Geometry check sheet. Reference: the model listing, model coordinates, mm. A direction names the side the tool comes from. Give positions to 0.01 mm unless a question says otherwise; leave off trailing zeros. Write each loop counter-clockwise with the first axis right and the second up, starting at its lowest first coordinate (ties: lowest second). Pieces come first, ordered by that corner, then holes.
(1) Tool access check on faces 1 (the flat face through (41.686, -9, 5)), 2 (the flat face through (70, 4.42, 5)), 3 (the flat face through (8.02, -22, 5)), 4 (the flat face through (0, -38.015, 5)). Record the directions out of +Z, -Z, +X, -X, +Y, -Y that give a thin tool (end or side, any length) a straight path to the whole face; none if there is none.
(2) Cross-section at C-C (x = 29). Record the boundary of the cut face in (y, z), and give its area (3 significant figures).
(3) Thickness scan on line 1 along X through (y, z) = (-44.5, 8.5); line 2 along Y through (x, z) = (39.5, 6.75); line 3 along Y through (x, z) = (54.5, 1.25). Record the ranges inside material, lowest first.
(4) Mould release check, pull along X, two halves, no side actions. Record for faces 5 (the flat face through (40, -17.929, 5)), 6 (the flat face through (15.282, -44, 4)), 7 (the flat face through (67.806, 16, 5)): +X half, -X half, draft (parallel to the pull), parting line (faces both ways), or undercut.
(5) Cross-section at A-A (y = -42). Record the boundary of the cut face in (x, z), and give its area (3 significant figures).
(6) Depth check by flat-ended pin: P1, Ø8, axis at x = 55.5, y = -3, coming from the +Z side; P2, Ø3.5, axis at x = 55.5, z = 5, coming from the -Y side; P3, Ø1.1, axis at x = -17, z = 2.5, coming from the +Y side; P4, Ø6, axis at x = 40, y = -37.5, coming from the +Z side. Enter the tip coordinate at first touch or a pass-through.
Autodesk Fusion 360 part; units mm, degrees
sketch "Dino" plane through (0, 0, 0) normal (0, 0, 1) x (1, 0, 0)
  line L0 (-25.8333, -18.1173) -> (-25.8333, -25.4727)
  line L1 (-25.8333, -25.4727) -> (-22.0613, -25.4727)
  line L2 (-22.0613, -25.4727) -> (-22.0613, -30.282)
  line L3 (-22.0613, -30.282) -> (-18.2893, -30.282)
  line L4 (-18.2893, -30.282) -> (-18.2893, -32.9224)
  line L5 (-18.2893, -32.9224) -> (-10.9339, -32.9224)
  line L6 (-10.9339, -32.9224) -> (-10.9339, -35.3742)
  line L7 (-10.9339, -35.3742) -> (-3.3899, -35.3742)
  line L8 (-3.3899, -35.3742) -> (-3.3899, -38.0146)
  line L9 (-3.3899, -38.0146) -> (4.2484, -38.0146)
  line L10 (4.2484, -38.0146) -> (4.2484, -47.9161)
  line L11 (4.2484, -47.9161) -> (11.5095, -47.9161)
  line L12 (11.5095, -47.9161) -> (11.5095, -40.3721)
  line L13 (11.5095, -40.3721) -> (15.2815, -40.3721)
  line L14 (15.2815, -40.3721) -> (15.2815, -47.9161)
  line L15 (15.2815, -47.9161) -> (26.5975, -47.9161)
  line L16 (26.5975, -40.3721) -> (30.0866, -40.3721)
  line L17 (30.0866, -40.3721) -> (30.0866, -47.9161)
  line L18 (30.0866, -47.9161) -> (37.9135, -47.9161)
  line L19 (37.9135, -47.9161) -> (37.9135, -40.3721)
  line L20 (37.9135, -40.3721) -> (41.4969, -40.3721)
  line L21 (41.4969, -40.3721) -> (41.4969, -47.9161)
  line L22 (41.4969, -47.9161) -> (48.9466, -47.9161)
  line L23 (48.9466, -47.9161) -> (48.9466, -33.0167)
  line L24 (48.9466, -33.0167) -> (52.2471, -33.0167)
  line L25 (52.2471, -33.0167) -> (52.2471, -27.8302)
  line L26 (52.2471, -27.8302) -> (56.5849, -27.8302)
  line L27 (56.5849, -27.8302) -> (56.5849, -15.194)
  line L28 (56.5849, -15.194) -> (52.2471, -15.194)
  line L29 (52.2471, -15.194) -> (52.2471, 4.4204)
  line L30 (52.2471, 4.4204) -> (56.5849, 4.4204)
  line L31 (56.5849, 4.4204) -> (56.5849, 1.8743)
  line L32 (56.5849, 1.8743) -> (67.8065, 1.8743)
  line L33 (67.8065, 1.8743) -> (67.8065, 4.4204)
  line L34 (67.8065, 4.4204) -> (71.5785, 4.4204)
  line L35 (71.5785, 4.4204) -> (71.5785, 14.6048)
  line L36 (71.5785, 14.6048) -> (67.8065, 14.6048)
  line L37 (67.8065, 14.6048) -> (67.8065, 17.1509)
  line L38 (67.8065, 17.1509) -> (64.1289, 17.1509)
  line L39 (64.1289, 17.1509) -> (64.1289, 19.5084)
  line L40 (64.1289, 19.5084) -> (45.1746, 19.5084)
  line L41 (45.1746, 19.5084) -> (45.1746, 17.1509)
  line L42 (45.1746, 17.1509) -> (41.6855, 17.1509)
  line L43 (41.6855, 17.1509) -> (41.6855, 14.5105)
  line L44 (41.6855, 14.5105) -> (38.1021, 14.5105)
  line L45 (38.1021, 14.5105) -> (38.1021, -0.4832)
  line L46 (38.1021, -0.4832) -> (41.6855, -0.4832)
  line L47 (41.6855, -0.4832) -> (41.6855, -17.9287)
  line L48 (41.6855, -17.9287) -> (38.1021, -17.9287)
  line L49 (38.1021, -17.9287) -> (38.1021, -20.5691)
  line L50 (38.1021, -20.5691) -> (34.2358, -20.5691)
  line L51 (34.2358, -20.5691) -> (34.2358, -17.9287)
  line L52 (34.2358, -17.9287) -> (15.4701, -17.9287)
  line L53 (15.4701, -17.9287) -> (15.4701, -20.5691)
  line L54 (15.4701, -20.5691) -> (8.0204, -20.5691)
  line L55 (8.0204, -20.5691) -> (8.0204, -23.1152)
  line L56 (8.0204, -23.1152) -> (4.0598, -23.1152)
  line L57 (4.0598, -23.1152) -> (4.0598, -25.2841)
  line L58 (4.0598, -25.2841) -> (0.2878, -25.2841)
  line L59 (0.2878, -25.2841) -> (0.2878, -27.6416)
  line L60 (0.2878, -27.6416) -> (-10.8396, -27.6416)
  line L61 (-10.8396, -27.6416) -> (-10.8396, -25.2841)
  line L62 (-10.8396, -25.2841) -> (-14.5173, -25.2841)
  line L63 (-14.5173, -25.2841) -> (-14.5173, -23.1152)
  line L64 (-14.5173, -23.1152) -> (-18.195, -23.1152)
  line L65 (-18.195, -23.1152) -> (-18.195, -20.3805)
  line L66 (-18.195, -20.3805) -> (-21.967, -20.3805)
  line L67 (-25.8333, -18.1173) -> (-22.002, -18.1173)
  line L68 (-22.002, -18.1173) -> (-21.967, -20.3805)
  line L69 (11.5095, -40.3721) -> (11.5095, -37.7886)
  line L70 (11.5095, -37.7886) -> (30.0797, -37.7886)
  line L71 (30.0797, -37.7886) -> (30.0866, -40.3721)
  line L72 (30.0866, -40.3721) -> (26.5975, -40.3721)
  line L73 (37.9135, -40.3721) -> (37.9135, -35.4027)
  line L74 (37.9135, -35.4027) -> (41.4793, -35.4027)
  line L75 (41.4793, -35.4027) -> (41.4793, -32.8357)
  line L76 (41.4793, -32.8357) -> (45.2799, -32.8357)
  line L77 (45.2799, -32.8357) -> (45.2799, -30.4315)
  line L78 (45.2799, -30.4315) -> (49.0411, -30.4315)
  line L79 (49.0411, -30.4315) -> (49.0411, 4.3785)
  line L80 (49.0411, 4.3785) -> (52.2471, 4.4204)
  line L81 (59.9748, 12.022) -> (59.9748, 9.3751)
  line L82 (59.9748, 9.3751) -> (64.1657, 9.3751)
  line L83 (64.1657, 9.3751) -> (64.1657, 12.0124)
  line L84 (64.1657, 12.0124) -> (59.9748, 12.022)
  line L85 (15.2815, -40.3721) -> (26.5975, -40.3721)
  line L86 (26.5975, -45.2558) -> (26.5975, -47.9161)
  line L87 (26.5975, -45.2558) -> (26.5975, -40.3721)
  line L88 (41.4969, -40.3721) -> (41.4969, -38)
  line L89 (41.4969, -38) -> (45.2217, -38)
  line L90 (45.2217, -38) -> (45.2217, -35.3158)
  line L91 (45.2217, -35.3158) -> (48.9466, -35.3158)
extrude "Extrude18" add sketch "Dino" along normal blind 10 contours L0 L1 L2 L3 L4 L5 L6 L7 L8 L9 L10 L11 L12 L17 L18 L19 L30 L31 L32 L33 L34 L35 L36 L37 L38 L39 L40 L41 L42 L43 L44 L45 L46 L47 L48 L49 L50 L51 L52 L53 L54 L55 L56 L57 L58 L59 L60 L61 L62 L63 L64 L65 L66 L67 L68 L69 L70 L71 L73 L74 L75 L76 L77 L78 L79 L80
extrude "Extrude19" add sketch "Dino" along normal blind 7.5 contours L13 L16 L69 L70 L71 L72 L85 | L20 L23 L24 L25 L26 L27 L28 L29 L73 L74 L75 L76 L77 L78 L79 L80 L88 L89 L90 L91
extrude "Extrude20" add sketch "Dino" along normal blind 7.49 contours L14 L15 L85 L86 L87 | L21 L22 L23 L88 L89 L90 L91
extrude "Extrude21" cut sketch "Dino" along normal blind 0.01 contours L20 L23 L24 L25 L26 L27 L28 L29 L73 L74 L75 L76 L77 L78 L79 L80 L88 L89 L90 L91
Reply:
1. face 1: +Z, -Z, -X
1. face 2: +Z, -Z, +X, -Y
1. face 3: +Z, -Z, +Y
1. face 4: +Z, -Z, -X, -Y
2. outline: (-40.37, 0) - (-17.93, 0) - (-17.93, 10) - (-37.79, 10) - (-37.79, 7.5) - (-40.37, 7.5) - close
2. area: 218 mm2
3. line 1: x = 4.25 to 11.51, 30.09 to 37.91
3. line 2: y = -40.37 to -17.93, -0.48 to 14.51
3. line 3: y = -27.83 to -15.19, 4.42 to 19.51
4. face 5: draft
4. face 6: undercut
4. face 7: +X half
5. outline: (4.25, 0) - (11.51, 0) - (11.51, 10) - (4.25, 10) - close; (15.28, 0) - (26.6, 0) - (26.6, 7.49) - (15.28, 7.49) - close; (30.09, 0) - (37.91, 0) - (37.91, 10) - (30.09, 10) - close; (41.5, 0) - (48.95, 0) - (48.95, 7.49) - (41.5, 7.49) - close
5. area: 291 mm2
6. P1: stops at z = 7.5
6. P2: stops at y = -27.83
6. P3: stops at y = -23.12
6. P4: stops at z = 10
